Geometry: final body of the model. Coordinates: model frame, mm. Face numbers are marked on the shaded views. A direction names the side the tool comes from. Give positions to 0.01 mm unless a question says otherwise; leave off trailing zeros. Order: outer loops, then holes, each group sorted by start corner. A loop starts at its lowest first (then second) coordinate and runs counter-clockwise, first axis right, second up. Notation, with made-up numbers: M 52,-6.5 L 63,-6.5 A18 ccw 63,21.5 Z; hole C 72,28 d10. An arc over 180 degrees is marked long. Write item = value, one per line. Start each with the question number.
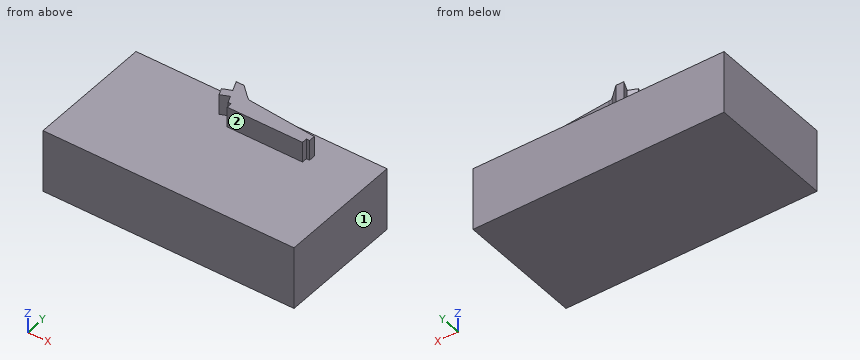
from build123d import *

# Parameters (mm, degrees)
SKETCH1_W      = 203.2
SKETCH1_H      = 101.6
EXTRUDE1_DEPTH = 50.8
EXTRUDE2_DEPTH = 16.51


with BuildPart() as part:
    # Sketch1 → Extrude1 (new body)
    with BuildSketch(Plane.XY):
        with Locations((101.6, 50.8)):
            Rectangle(SKETCH1_W, SKETCH1_H)
    extrude(amount=EXTRUDE1_DEPTH)

    # Sketch20 → Extrude2 (add)
    with BuildSketch(Plane.XY.offset(50.8)):
        with BuildLine():
            ThreePointArc((98.73765298, 90.37654578), (100.476619995, 89.229944151), (102.493050685, 88.707728828))
            Line((102.493050685, 88.707728828), (157.48, 83.82))
            Line((157.48, 83.82), (157.48, 78.74))
            Line((157.48, 78.74), (154.94, 78.74))
            Line((154.94, 78.74), (154.94, 74.422))
            Line((154.94, 74.422), (93.98, 74.422))
            Line((93.98, 74.422), (93.98, 78.74))
            Line((93.98, 78.74), (91.44, 78.74))
            Line((91.44, 78.74), (89.009960204, 84.606635031))
            Line((89.009960204, 84.606635031), (81.969998167, 81.690587277))
            Line((81.969998167, 81.690587277), (79.539958371, 87.557222308))
            Line((79.539958371, 87.557222308), (86.579920409, 90.473270063))
            Line((86.579920409, 90.473270063), (83.023180413, 99.06))
            Line((83.023180413, 99.06), (89.373180413, 99.06))
            Line((89.373180413, 99.06), (98.73765298, 90.37654578))
        make_face()
    extrude(amount=EXTRUDE2_DEPTH)


solid = part.part
1) Cut plane B-B (z = 57.5). Return loops of the section in (x, y), plus the area to 3 significant figures.
2) Cut plane A-A (x = 134.5). Return loops of the section in (y, z), plus the area to 3 significant figures.
3) Pin query (flat end, axial travel): pin 1 Ø0.8 at (x, z) = (93, 62) entering from -Y; pin 2 Ø4.5 at (y, z) = (77, 63) entering from +X; pin 3 Ø2 at (y, z) = (77, 58.5) entering from -X. Return the tip coordinate at first contact, or that it passes through.
4) Cut plane C-C (y = 22). Return loops of the section in (x, z), plus the area to 3 significant figures.
5) Ray query, L1, parallel to Z at x = 40.5, y = 74; L2, parallel to X at y = 80.5, z = 52.5. Return the intervals inside material, ascending.
6) Access query for the marked faces 1 and 2. Directions: +Z, -Z, +X, -X, +Y, -Y. A direction counts if a zero-diameter tool reaches every point of the face in a straight line with its end or side. Return the directions, or none.
7) Cut plane D-D (y = 94.5). Return loops of the section in (x, z).
Reply:
q1.outline = M 79.54,87.56 L 81.97,81.69 L 89.01,84.61 L 91.44,78.74 L 93.98,78.74 L 93.98,74.42 L 154.94,74.42 L 154.94,78.74 L 157.48,78.74 L 157.48,83.82 L 102.49,88.71 A6.35 cw 98.74,90.38 L 89.37,99.06 L 83.02,99.06 L 86.58,90.47 Z
q1.area = 958 mm²
q2.outline = M 0,0 L 101.6,0 L 101.6,50.8 L 85.86,50.8 L 85.86,67.31 L 74.42,67.31 L 74.42,50.8 L 0,50.8 Z
q2.area = 5,350 mm²
q3.pin_1 = 78.74
q3.pin_2 = 157.48
q3.pin_3 = 93.98
q4.outline = M 0,0 L 203.2,0 L 203.2,50.8 L 0,50.8 Z
q4.area = 10,300 mm²
q5.L1 = 0 to 50.8
q5.L2 = 90.71 to 157.48
q6.face_1 = +Z, -Z, +X, +Y, -Y
q6.face_2 = +Z, +X, -X, -Y
q7.outline = M 0,0 L 203.2,0 L 203.2,50.8 L 94.29,50.8 L 94.29,67.31 L 84.91,67.31 L 84.91,50.8 L 0,50.8 Z
